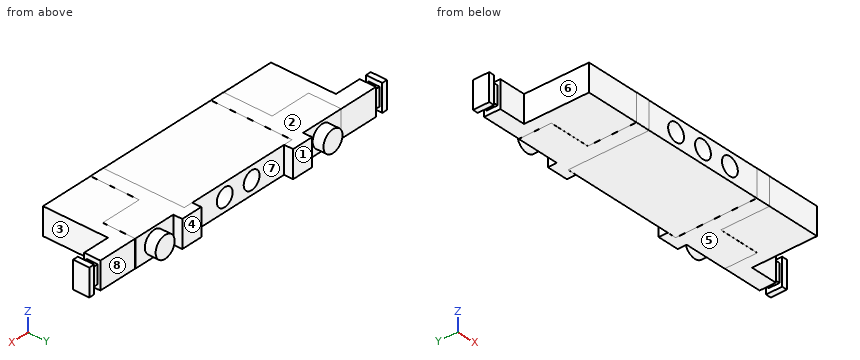
Autodesk Inventor part; units mm, degrees
ref_plane "Work Plane1" through (0, 0, 4.7625) normal (0, 0, 1) x (1, 0, 0)
ref_plane "YZ Plane" through (0, 0, 0) normal (1, 0, 0) x (0, 1, 0)
ref_plane "XZ Plane" through (0, 0, 0) normal (0, 1, 0) x (-1, 0, 0)
sketch "Sketch1" plane through (0, 0, 0) normal (0, 0, 1) x (1, 0, 0)
  line L0 (52.6803, 14.9225) -> (52.6803, -13.6525)
  line L1 (52.6803, -13.6525) -> (-38.7597, -13.6525)
  line L2 (-38.7597, -13.6525) -> (-38.7597, 14.9225)
  line L3 (-19.0747, 18.0975) -> (-11.4547, 18.0975)
  line L4 (-11.4547, 18.0975) -> (-11.4547, 14.9225)
  line L5 (-19.0747, 14.9225) -> (-19.0747, 18.0975)
  line L6 (25.3753, 18.0975) -> (32.9953, 18.0975)
  line L7 (32.9953, 18.0975) -> (32.9953, 14.9225)
  line L8 (25.3753, 14.9225) -> (25.3753, 18.0975)
  line L9 (32.9953, 14.9225) -> (52.6803, 14.9225)
  line L10 (-38.7597, 14.9225) -> (-19.0747, 14.9225)
  line L11 (-11.4547, 14.9225) -> (25.3753, 14.9225)
  point P0 (0, 0)
  dimension "d0" = 28.575
  dimension "d1" = 91.44
  dimension "d2" = 7.62
  dimension "d3" = 7.62
  dimension "d4" = 3.175
  dimension "d5" = 3.175
  dimension "d6" = 3.175
  dimension "d7" = 3.175
  dimension "d8" = 19.685
  dimension "d9" = 19.685
  dimension "d10" = 36.83
extrude "Extrusion1" add sketch "Sketch1" along normal blind 9.525
sketch "Sketch2" plane through (0, 0, 9.525) normal (0, 0, 1) x (1, 0, 0)
  line L0 (-38.7597, 14.9225) -> (-19.0747, 14.9225)
  line L1 (52.6803, -13.6525) -> (-38.7597, -13.6525)
  line L2 (32.9953, 14.9225) -> (52.6803, 14.9225)
  line L3 (32.9953, 18.0975) -> (32.9953, 14.9225)
  line L4 (25.3753, 18.0975) -> (32.9953, 18.0975)
  line L5 (25.3753, 14.9225) -> (25.3753, 18.0975)
  line L6 (-11.4547, 18.0975) -> (-11.4547, 14.9225)
  line L7 (-19.0747, 18.0975) -> (-11.4547, 18.0975)
  line L8 (-19.0747, 14.9225) -> (-19.0747, 18.0975)
  line L9 (-11.4547, 14.9225) -> (-14.6297, 14.9225)
  line L10 (-14.6297, 14.9225) -> (-14.6297, -13.6525)
  line L11 (25.3753, 14.9225) -> (28.5503, 14.9225)
  line L12 (28.5503, 14.9225) -> (28.5503, -13.6525)
  line L13 (33.6303, -13.6525) -> (33.6303, 3.4925)
  line L14 (33.6303, 3.4925) -> (48.2353, 3.4925)
  line L15 (48.2353, 3.4925) -> (48.2353, 14.9225)
  line L16 (-19.7097, -13.6525) -> (-19.7097, 3.4925)
  line L17 (-19.7097, 3.4925) -> (-34.3147, 3.4925)
  line L18 (-34.3147, 3.4925) -> (-34.3147, 14.9225)
  point P0 (0, 0)
  dimension "d13" = 3.175
  dimension "d14" = 3.175
  dimension "d15" = 5.08
  dimension "d16" = 5.08
  dimension "d17" = 19.685
  dimension "d18" = 19.685
  dimension "d19" = 11.43
  dimension "d20" = 11.43
extrude "Extrusion2" add sketch "Sketch2" along normal blind 0.0254
sketch "Sketch3" plane through (0, 0, 0) normal (0, 0, -1) x (-1, 0, 0)
  line L0 (19.0747, 14.9225) -> (38.7597, 14.9225)
  line L1 (19.0747, 18.0975) -> (19.0747, 14.9225)
  line L2 (11.4547, 18.0975) -> (19.0747, 18.0975)
  line L3 (11.4547, 14.9225) -> (11.4547, 18.0975)
  line L4 (-25.3753, 18.0975) -> (-25.3753, 14.9225)
  line L5 (-32.9953, 18.0975) -> (-25.3753, 18.0975)
  line L6 (-32.9953, 14.9225) -> (-32.9953, 18.0975)
  line L7 (-52.6803, 14.9225) -> (-32.9953, 14.9225)
  line L8 (38.7597, -13.6525) -> (-52.6803, -13.6525)
  line L9 (-28.5503, -13.6525) -> (-28.5503, 14.9225)
  line L10 (-28.5503, 14.9225) -> (-25.3753, 14.9225)
  line L11 (-48.2353, 14.9225) -> (-48.2353, 3.4925)
  line L12 (-48.2353, 3.4925) -> (-33.6303, 3.4925)
  line L13 (-33.6303, 3.4925) -> (-33.6303, -13.6525)
  line L14 (14.6297, 14.9225) -> (14.6297, -13.6525)
  line L15 (11.4547, 14.9225) -> (14.6297, 14.9225)
  line L16 (34.3147, 3.4925) -> (34.3147, 14.9225)
  line L17 (19.7097, 3.4925) -> (34.3147, 3.4925)
  line L18 (19.7097, -13.6525) -> (19.7097, 3.4925)
  point P0 (0, 0)
extrude "Extrusion3" add sketch "Sketch3" along normal blind 0.0254
sketch "Sketch4" plane through (-38.7597, -13.6525, 0) normal (0, -1, 0) x (1, 0, 0)
  line L0 (72.39, 9.5504) -> (67.31, 9.5504)
  line L1 (67.31, 9.525) -> (67.31, 9.5504)
  line L2 (67.31, -0.0254) -> (72.39, -0.0254)
  line L3 (72.39, 0) -> (72.39, -0.0254)
  line L4 (19.685, -0.0254) -> (4.445, -0.0254)
  line L5 (27.305, -0.0254) -> (19.685, -0.0254)
  line L6 (24.13, -0.0254) -> (27.305, -0.0254)
  line L7 (19.05, -0.0254) -> (24.13, -0.0254)
  line L8 (4.445, -0.0254) -> (19.05, -0.0254)
  line L9 (72.39, 0) -> (72.39, 9.5504)
  line L10 (24.13, -0.0254) -> (24.13, 9.5504)
  line L11 (19.05, -0.0254) -> (19.05, 9.525)
  line L12 (67.31, -0.0254) -> (67.31, 9.525)
  line L13 (91.44, 0) -> (91.44, 9.525)
  line L14 (24.13, 0) -> (19.05, 0)
  line L15 (19.05, 9.5504) -> (24.13, 9.525)
  line L16 (24.13, 0) -> (19.05, 0)
  line L17 (19.05, 0) -> (19.05, 9.5504)
  line L18 (19.05, 9.5504) -> (24.13, 9.5504)
  line L19 (24.13, 9.5504) -> (24.13, 0)
  point P0 (38.7597, 0)
extrude "Extrusion4" add sketch "Sketch4" along normal blind 0.0254 contours L9 L3 L2 L12 L1 L0 | L11 L17 L15 L10 L14 | L15 L18 L10
sketch "Sketch5" plane through (52.6803, 14.9225, 9.525) normal (0, 1, 0) x (1, 0, 0)
  line L0 (-4.445, 9.5504) -> (-19.685, 9.5504)
  line L1 (-19.685, -0.0254) -> (-4.445, -0.0254)
  line L2 (-64.135, 0) -> (-27.305, 0)
  line L3 (-27.305, 9.525) -> (-27.305, 0)
  line L4 (-27.305, 9.525) -> (-64.135, 9.525)
  line L5 (-64.135, 9.525) -> (-64.135, 0)
  line L6 (-91.44, 0) -> (-86.995, 0)
  line L7 (-86.995, 0) -> (-86.995, -0.0254)
  line L8 (-86.995, -0.0254) -> (-71.755, -0.0254)
  line L9 (-71.755, 9.5504) -> (-71.755, -0.0254)
  line L10 (-71.755, 9.5504) -> (-86.995, 9.5504)
  line L11 (-86.995, 9.525) -> (-86.995, 9.5504)
  line L12 (-86.995, 9.525) -> (-91.44, 9.525)
  line L13 (-91.44, 9.525) -> (-91.44, 0)
  line L14 (-71.755, 9.5504) -> (-71.755, -0.0254)
  line L15 (-27.305, 9.5504) -> (-27.305, -0.0254)
  line L16 (-19.685, 9.5504) -> (-19.685, -0.0254)
  line L17 (-64.135, 9.5504) -> (-64.135, -0.0254)
  line L18 (-4.445, 9.5504) -> (-4.445, -0.0254)
  line L19 (-86.995, -0.0254) -> (-86.995, 9.525)
  point P0 (-52.6803, 9.525)
extrude "Extrusion5" add sketch "Sketch5" along normal blind 0.0254 contours L18 L1 L16 L0 | L19 L11 L10 L9 L8 L7
sketch "Sketch6" plane through (0, 0, 0) normal (0, 0, -1) x (-1, 0, 0)
  line L0 (-52.6803, -13.6525) -> (-52.6803, 14.9225)
  line L1 (19.7097, 3.4925) -> (19.7097, -13.6525)
  line L2 (38.7597, -13.6525) -> (19.7097, -13.6525)
  line L3 (38.7597, 14.9225) -> (38.7597, -13.6525)
  line L4 (34.3147, 14.9225) -> (38.7597, 14.9225)
  line L5 (34.3147, 14.9225) -> (34.3147, 3.4925)
  line L6 (34.3147, 3.4925) -> (19.7097, 3.4925)
  line L7 (-62.2053, 14.9225) -> (-52.6803, 14.9225)
  line L8 (-52.6803, 14.9225) -> (-52.6803, 9.2075)
  line L9 (-52.6803, 9.2075) -> (-62.2053, 9.2075)
  line L10 (-62.2053, 9.2075) -> (-62.2053, 14.9225)
  line L11 (38.7597, 14.9225) -> (48.2847, 14.9225)
  line L12 (48.2847, 14.9225) -> (48.2847, 9.2075)
  line L13 (48.2847, 9.2075) -> (38.7597, 9.2075)
  line L14 (38.7597, 9.2075) -> (38.7597, 14.9225)
  point P0 (0, 0)
  dimension "d29" = 9.525
  dimension "d30" = 9.525
  dimension "d31" = 5.715
  dimension "d32" = 5.715
extrude "Extrusion6" add sketch "Sketch6" against normal blind 9.525 contours L9 L10 L7 L0 | L3 L11 L12 L13
ref_plane "Work Plane1" through (0, 0, 4.7625) normal (0, 0, 1) x (1, 0, 0)
sketch "Sketch7" plane through (0, 0, 4.7625) normal (0, 0, 1) x (1, 0, 0)
  line L0 (-19.7097, 3.4925) -> (-19.7097, -13.6525)
  line L1 (-38.7597, -13.6525) -> (-19.7097, -13.6525)
  line L2 (-38.7597, 9.2075) -> (-38.7597, -13.6525)
  line L3 (-38.7597, 9.2075) -> (-48.2847, 9.2075)
  line L4 (-48.2847, 9.2075) -> (-48.2847, 14.9225)
  line L5 (-34.3147, 14.9225) -> (-48.2847, 14.9225)
  line L6 (-34.3147, 14.9225) -> (-34.3147, 3.4925)
  line L7 (-34.3147, 3.4925) -> (-19.7097, 3.4925)
  line L8 (48.2353, 3.4925) -> (48.2353, 14.9225)
  line L9 (48.2353, 14.9225) -> (62.2053, 14.9225)
  line L10 (62.2053, 14.9225) -> (62.2053, 9.2075)
  line L11 (62.2053, 9.2075) -> (52.6803, 9.2075)
  line L12 (52.6803, -13.6525) -> (52.6803, 9.2075)
  line L13 (33.6303, -13.6525) -> (52.6803, -13.6525)
  line L14 (33.6303, -13.6525) -> (33.6303, 3.4925)
  line L15 (33.6303, 3.4925) -> (48.2353, 3.4925)
  line L16 (-48.2847, 13.97) -> (-50.8247, 13.97)
  line L17 (-50.8247, 13.97) -> (-50.8247, 10.16)
  line L18 (-50.8247, 10.16) -> (-48.2847, 10.16)
  line L19 (-48.2847, 10.16) -> (-48.2847, 13.97)
  line L20 (62.2053, 13.97) -> (64.7453, 13.97)
  line L21 (64.7453, 13.97) -> (64.7453, 10.16)
  line L22 (64.7453, 10.16) -> (62.2053, 10.16)
  line L23 (62.2053, 10.16) -> (62.2053, 13.97)
  point P0 (0, 0)
  dimension "d36" = 2.54
  dimension "d37" = 2.54
  dimension "d38" = 3.81
  dimension "d39" = 3.81
  dimension "d40" = 0.9525
  dimension "d41" = 0.9525
  dimension "d42" = 0.9525
extrude "Extrusion7" add sketch "Sketch7" along normal mid plane 6.35 contours L4 L18 L17 L16 | L20 L21 L22 L10
sketch "Sketch8" plane through (0, 0, 4.7625) normal (0, 0, 1) x (1, 0, 0)
  line L0 (-48.2847, 13.97) -> (-48.2847, 10.16)
  line L1 (-50.8247, 13.97) -> (-48.2847, 13.97)
  line L2 (-50.8247, 10.16) -> (-50.8247, 13.97)
  line L3 (-48.2847, 10.16) -> (-50.8247, 10.16)
  line L4 (62.2053, 13.97) -> (64.7453, 13.97)
  line L5 (62.2053, 10.16) -> (62.2053, 13.97)
  line L6 (64.7453, 10.16) -> (62.2053, 10.16)
  line L7 (64.7453, 13.97) -> (64.7453, 10.16)
  line L8 (-52.7297, 14.9225) -> (-50.8247, 14.9225)
  line L9 (-50.8247, 14.9225) -> (-50.8247, 9.2075)
  line L10 (-50.8247, 9.2075) -> (-52.7297, 9.2075)
  line L11 (-52.7297, 9.2075) -> (-52.7297, 14.9225)
  line L12 (64.7453, 14.9225) -> (66.6503, 14.9225)
  line L13 (66.6503, 14.9225) -> (66.6503, 9.2075)
  line L14 (66.6503, 9.2075) -> (64.7453, 9.2075)
  line L15 (64.7453, 9.2075) -> (64.7453, 14.9225)
  line L16 (48.2353, 14.9225) -> (62.2053, 14.9225)
  line L17 (62.2053, 9.2075) -> (52.6803, 9.2075)
  line L18 (-38.7597, 9.2075) -> (-48.2847, 9.2075)
  line L19 (-48.2847, 14.9225) -> (-34.3147, 14.9225)
  point P0 (0, 0)
  dimension "d45" = 0
  dimension "d46" = 0
  dimension "d47" = 0
  dimension "d48" = 0
  dimension "d49" = 1.905
  dimension "d50" = 5.715
  dimension "d51" = 0
  dimension "d52" = 1.905
  dimension "d53" = 0
extrude "Extrusion8" add sketch "Sketch8" along normal mid plane 9.525 contours L2 L9 L10 L11 L8 | L15 L12 L13 L14 L7
sketch "Sketch9" plane through (52.6803, 14.9479, 9.525) normal (0, 1, 0) x (1, 0, 0)
  line L0 (-4.445, 9.5504) -> (-4.445, -0.0254)
  line L1 (-19.685, 9.5504) -> (-4.445, 9.5504)
  line L2 (-19.685, -0.0254) -> (-19.685, 9.5504)
  line L3 (-4.445, -0.0254) -> (-19.685, -0.0254)
  circle A0 centre (-12.065, 4.7625) radius 3.81
  circle A1 centre (-79.375, 4.7625) radius 3.81
  point P0 (-52.6803, 9.525)
  dimension "d56" = 7.62
  dimension "d57" = 7.62
extrude "Extrusion9" add sketch "Sketch9" along normal blind 3.81 contours A0 | A1
sketch "Sketch10" plane through (-14.6297, -13.6525, 9.525) normal (0, -1, 0) x (1, 0, 0)
  line L0 (43.18, -9.525) -> (43.18, 0)
  line L1 (0, 0) -> (0, -9.525)
  circle A0 centre (10.795, -4.7625) radius 3.175
  circle A1 centre (21.59, -4.7625) radius 3.175
  circle A2 centre (32.385, -4.7625) radius 3.175
  point P0 (14.6297, -9.525)
  dimension "d60" = 6.35
  dimension "d61" = 10.795
  dimension "d62" = 10.795
  dimension "d63" = 10.795
  dimension "d64" = 10.795
extrude "Extrusion10" cut sketch "Sketch10" against normal blind 10.16
sketch "Sketch11" plane through (-11.4547, 14.9225, 9.525) normal (0, 1, 0) x (1, 0, 0)
  line L0 (36.83, 9.525) -> (36.83, 0)
  line L1 (0, 9.525) -> (0, 0)
  circle A0 centre (23.8125, 4.7625) radius 3.175
  circle A1 centre (13.0175, 4.7625) radius 3.175
  line L2 (23.8125, 4.7625) -> (36.83, 4.7625)
  line L3 (13.0175, 4.7625) -> (0, 4.7625)
  point P0 (11.4547, 9.525)
  dimension "d67" = 6.35
  dimension "d68" = 10.795
extrude "Extrusion11" cut sketch "Sketch11" against normal blind 10.16
sketch "Sketch12" plane through (0, 0, 9.525) normal (0, 0, 1) x (1, 0, 0)
  line L0 (-11.4547, 14.9225) -> (25.3753, 14.9225)
  line L1 (-14.6297, 14.9225) -> (-14.6297, -13.6525)
  line L2 (28.5503, -13.6525) -> (-14.6297, -13.6525)
  line L3 (-10.8197, -9.525) -> (-10.8197, 10.795) construction
  line L4 (-10.8197, 10.795) -> (-6.9164, 10.795) construction
  line L5 (-6.9164, 10.795) -> (-6.9164, -9.525) construction
  line L6 (-6.9164, -9.525) -> (-10.8197, -9.525) construction
  point P0 (0, 0)
  dimension "d72" = 20.32
  dimension "d84" = 3.81
  dimension "d85" = 4.1275
  dimension "d86" = 4.1275
decal "Decal1"
properties part number "Festo Valve 1764"
The listing builds one solid part. Answer for the finished solid, in the listing's coordinates (mm). Face numbers are marked on the shaded views. A direction names the side the tool comes from. Coordinates: 2 decimals unless noted, no trailing zeros. Write each loop counter-clockwise with the first axis right and the second up, starting at its lowest first coordinate (ties: lowest second). Pieces come first, ordered by that corner, then holes. Notation, with made-up numbers: (65, 55) - (96, 55) arc R5 ccw to (96, 60) - close; hole circle Ø8 at (15, 70). An arc over 180 degrees is marked (long way). One line per item, written item: value.
1) Each of these flat-tipped pins is pushed along its axis until it touches: pin 1 Ø1 at (x, y) = (65.5, 12.5) entering from +Z (3 decimals); pin 2 Ø1.3 at (x, y) = (-50, 12) entering from -Z; pin 3 Ø3 at (x, z) = (16.5, 4.5) entering from -Y. Where does it stop, or does it pass through?
Geometry check:
pin 1: stops at z = 9.525
pin 2: stops at z = 1.59
pin 3: stops at y = -3.49
2) Find section D-D (x = 18.5). Give the vertices of the cut face in (y, z) (1 decimal), and give its area (3 significant figures).
Geometry check:
outline: (-13.7, 0) - (14.9, 0) - (14.9, 9.5) - (-13.7, 9.5) - (-13.7, 7.8) - (-3.5, 7.8) - (-3.5, 1.7) - (-13.7, 1.7) - close
area: 209 mm2
3) A tool of negligible diameter and unlimited length cuts with its end or side. For the marked faces 5, 6, 7 and 8, from which of +Z, -Z, +X, -X, +Y, -Y can it reach the whole face along a straight path? Write none if from no direction.
Geometry check:
face 5: -Z, +X, -X, +Y, -Y
face 6: +Z, -Z, -X, -Y
face 7: +Z, -Z, +Y
face 8: +Z, -Z, +X, +Y
4) For a pull along X with two mould halves and no side action, classify the marked faces 1, 2, 3 and 4 as pulls with the +X half, pulls with the -X half, needs draft (parallel to the pull), parting line crosses it, or undercut.
Geometry check:
face 1: undercut
face 2: needs draft
face 3: pulls with the +X half
face 4: undercut
5) Find section A-A (y = 8). Count the separate pieces of the cut face and the enclosed holes in it, and give its area (3 significant figures).
Geometry check:
separate pieces: 1
enclosed holes: 2
area: 810 mm2
6) Consider line 1 along X through (y, z) = (14, 6.75); line 2 along X through (y, z) = (5, 2); line 3 along Z through (x, y) = (37, -1) (3 decimals). Determine where each line is inside the solid, lowest interval first. Write a range as from..to.
Geometry check:
line 1: x = -52.73..-50.82, -48.28..-0.91, 4.04..9.88, 14.83..62.21, 64.75..66.65
line 2: x = -38.76..0, 3.13..10.79, 13.92..52.68
line 3: z = 0..9.525
